Geometry check sheet. Reference: the model listing, model coordinates, mm. A direction names the side the tool comes from. Give positions to 0.01 mm unless a question says otherwise; leave off trailing zeros. Write each loop counter-clockwise with the first axis right and the second up, starting at its lowest first coordinate (ties: lowest second). Pieces come first, ordered by that corner, then holes. Notation, with made-up numbers: M -11.5,-20.75 L 13.5,-20.75 A16 cw 13.5,9.25 Z; hole C 56,77 d9. An arc over 180 degrees is marked long. Write each question's results on one line, items separated by ' | '.
```python
from build123d import *

# Parameters (mm, degrees)
SKETCH1_W           = 60
SKETCH1_H           = 50
BOSS_EXTRUDE1_DEPTH = 50
SKETCH2_W           = 20
SKETCH2_H           = 10
CUT_EXTRUDE1_DEPTH  = 50
SKETCH3_W           = 20
SKETCH3_H           = 20
CUT_EXTRUDE2_DEPTH  = 20
SKETCH4_W           = 40
SKETCH4_H           = 10
CUT_EXTRUDE3_DEPTH  = 30
SKETCH5_W           = 20
SKETCH5_H           = 20
CUT_EXTRUDE4_DEPTH  = 10
SKETCH6_W           = 20
SKETCH6_H           = 20
CUT_EXTRUDE5_DEPTH  = 10
SKETCH8_W           = 40
SKETCH8_H           = 10
BOSS_EXTRUDE2_DEPTH = 10
SKETCH9_W           = 20
SKETCH9_H           = 40
CUT_EXTRUDE6_DEPTH  = 20
SKETCH10_W          = 20
SKETCH10_H          = 20
CUT_EXTRUDE7_DEPTH  = 20


with BuildPart() as part:
    # Sketch1 → Boss-Extrude1 (new body)
    with BuildSketch(Plane.XY):
        with Locations((30, 25)):
            Rectangle(SKETCH1_W, SKETCH1_H)
    extrude(amount=BOSS_EXTRUDE1_DEPTH)

    # Sketch2 → Cut-Extrude1 (cut)
    with BuildSketch(Plane.XY.offset(50)):
        with Locations((10, 45)):
            Rectangle(SKETCH2_W, SKETCH2_H)
    extrude(amount=-CUT_EXTRUDE1_DEPTH, mode=Mode.SUBTRACT)

    # Sketch3 → Cut-Extrude2 (cut)
    with BuildSketch(Plane.XY.offset(50)):
        with Locations((10, 30)):
            Rectangle(SKETCH3_W, SKETCH3_H)
    extrude(amount=-CUT_EXTRUDE2_DEPTH, mode=Mode.SUBTRACT)

    # Sketch4 → Cut-Extrude3 (cut)
    with BuildSketch(Plane.XY.offset(50)):
        with Locations((40, 45)):
            Rectangle(SKETCH4_W, SKETCH4_H)
    extrude(amount=-CUT_EXTRUDE3_DEPTH, mode=Mode.SUBTRACT)

    # Sketch5 → Cut-Extrude4 (cut)
    with BuildSketch(Plane.XY.offset(30)):
        with Locations((10, 30)):
            Rectangle(SKETCH5_W, SKETCH5_H)
    extrude(amount=-CUT_EXTRUDE4_DEPTH, mode=Mode.SUBTRACT)

    # Sketch6 → Cut-Extrude5 (cut)
    with BuildSketch(Plane.XY.offset(50)):
        with Locations((10, 10)):
            Rectangle(SKETCH6_W, SKETCH6_H)
    extrude(amount=-CUT_EXTRUDE5_DEPTH, mode=Mode.SUBTRACT)

    # Sketch8 → Boss-Extrude2 (add)
    with BuildSketch(Plane.XY.offset(20)):
        with Locations((40, 45)):
            Rectangle(SKETCH8_W, SKETCH8_H)
    extrude(amount=BOSS_EXTRUDE2_DEPTH)

    # Sketch9 → Cut-Extrude6 (cut)
    with BuildSketch(Plane(origin=(0, 0, 0), x_dir=(-1, 0, 0), z_dir=(0, -1, 0))):
        with Locations((-50, -20)):
            Rectangle(SKETCH9_W, SKETCH9_H)
    extrude(amount=-CUT_EXTRUDE6_DEPTH, mode=Mode.SUBTRACT)

    # Sketch10 → Cut-Extrude7 (cut)
    with BuildSketch(Plane(origin=(0, 0, 0), x_dir=(-1, 0, 0), z_dir=(0, 0, -1))):
        with Locations((-50, 30)):
            Rectangle(SKETCH10_W, SKETCH10_H)
    extrude(amount=-CUT_EXTRUDE7_DEPTH, mode=Mode.SUBTRACT)


solid = part.part
```
Q1. Section check D-D (x = 7). Enter the section's corners in (y, z), then the cut area to 3 significant figures.
Answer key:
outline: M 0,0 L 40,0 L 40,20 L 20,20 L 20,40 L 0,40 Z | area: 1,200 mm2
Q2. Section check C-C (x = 51). Enter the section's corners in (y, z).
Answer key:
outline: M 0,40 L 20,40 L 20,20 L 40,20 L 40,0 L 50,0 L 50,30 L 40,30 L 40,50 L 0,50 Z
Q3. Material ranges on probe 1 along Z at (x, y) = (35, 44); probe 2 along X at (y, z) = (24, 7), recorded low to high. Write a range as [from, to].
Answer key:
probe 1: z = [0, 30] | probe 2: x = [0, 40]
Q4. Section check B-B (z = 32). Enter the section's corners in (x, y).
Answer key:
outline: M 0,0 L 40,0 L 40,20 L 60,20 L 60,40 L 20,40 L 20,20 L 0,20 Z
Q5. Depth check by flat-ended pin: P1, Ø5, axis at x = 10, z = 18.5, coming from the +Y side; P2, Ø16, axis at x = 54, z = 30.5, coming from the -Y side; P3, Ø4, axis at x = 45.5, y = 14, coming from the -Z side. Enter the tip coordinate at first touch or a pass-through.
Answer key:
P1: stops at y = 40 | P2: stops at y = 20 | P3: stops at z = 40
Q6. Access from +Z, -Z, +X, -X, +Y, -Y to the whole of each face (thin tool, end or side, straight path). Record for faces 1 (the face through (40, 45, 30)), 2 (the face through (10, 30, 20)), 3 (the face through (10, 40, 10)), 4 (the face through (50, 30, 20)), 5 (the face through (10, 10, 40)).
Answer key:
face 1: +Z, +X, -X, +Y | face 2: +Z, -X, +Y | face 3: +Z, -Z, -X, +Y | face 4: -Z, +X, -Y | face 5: +Z, -X, +Y, -Y
Q7. Section check A-A (y = 8). Enter the section's corners in (x, z).
Answer key:
outline: M 0,0 L 40,0 L 40,40 L 60,40 L 60,50 L 20,50 L 20,40 L 0,40 Z
